Read the model definition and answer for the solid it produces. Units are mm, in the model's axes. Face numbers are marked on the shaded views. A direction names the side the tool comes from. Coordinates: 2 decimals unless noted, no trailing zeros. Loops run counter-clockwise (first coordinate to the right, second up) from the corner with the lowest first, then second, coordinate; pieces in that order, holes last.
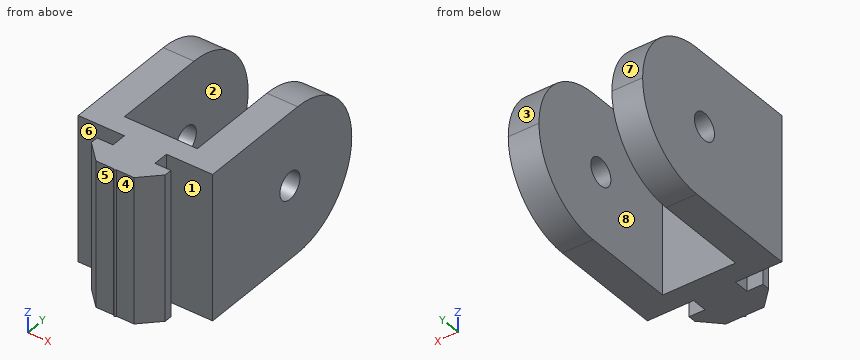
from build123d import *

# Parameters (mm, degrees)
SKETCH1_W           = 150
SKETCH1_H           = 70
BOSS_EXTRUDE1_DEPTH = 10
SKETCH2_W           = 18
SKETCH2_H           = 70
BOSS_EXTRUDE2_DEPTH = 80
FILLET1_R           = 35
SKETCH3_R           = 6.5
CUT_EXTRUDE1_DEPTH  = 164.102034121
RIB1_REACH          = 134.904
SKETCH5_WALL_W      = 321.142477346
SKETCH5_WALL_H      = 40
SKETCH7_W           = 43.830511012
SKETCH7_H           = 10.028409091
CUT_EXTRUDE2_DEPTH  = 80
SCALE1_SCALE        = 0.31
BOSS_EXTRUDE4_DEPTH = 21.7
CUT_EXTRUDE5_REACH  = 46.882
SKETCH11_W          = 1.005
SKETCH11_H          = 10.85
SKETCH11_H_2        = 13.95


with BuildPart() as part:
    # Sketch1 → Boss-Extrude1 (new body)
    with BuildSketch(Plane(origin=(0, 0, 0), x_dir=(1, 0, 0), z_dir=(0, 1, 0))):
        with Locations((14.225473782, -5.028409091)):
            Rectangle(SKETCH1_W, SKETCH1_H)
    extrude(amount=BOSS_EXTRUDE1_DEPTH)

    # Sketch2 → Boss-Extrude2 (add)
    with BuildSketch(Plane(origin=(0, 10, 0), x_dir=(1, 0, 0), z_dir=(0, 1, 0))):
        with Locations((-31.774526218, -5.028409091)):
            Rectangle(SKETCH2_W, SKETCH2_H)
        with Locations((21.225473782, -5.028409091)):
            Rectangle(SKETCH2_W, SKETCH2_H)
    extrude(amount=BOSS_EXTRUDE2_DEPTH)

    # Fillet1
    fillet1_edges = [part.edges().sort_by_distance(p)[0] for p in [
        (21.225473782, 90, 40.028409091),
        (21.225473782, 90, -29.971590909),
        (-31.774526218, 90, -29.971590909),
        (-31.774526218, 90, 40.028409091),
    ]]
    fillet(fillet1_edges, radius=FILLET1_R - 0.0001)  # a hair under: the kernel refuses the full size

    # Sketch3 → Cut-Extrude1 (cut, through all)
    with BuildSketch(Plane.ZY.offset(40.774526218)):
        with Locations((5.212032143, 50)):
            Circle(SKETCH3_R)
    extrude(amount=-CUT_EXTRUDE1_DEPTH, mode=Mode.SUBTRACT)

    # Sketch5 wall → Rib1 (add, up to next)
    with BuildSketch(Plane(origin=(52.140729288, 25.194278726, 0), x_dir=(0.821802771323, -0.569772064116, 0), z_dir=(0.569772064116, 0.821802771323, 0)), mode=Mode.PRIVATE) as rib1_sk1:
        Rectangle(SKETCH5_WALL_W, SKETCH5_WALL_H)
    rib1_tool1 = extrude(rib1_sk1.sketch, amount=-RIB1_REACH, mode=Mode.PRIVATE) - part.part
    add(rib1_tool1.solids().sort_by_distance((52.140729288, 25.194278726, 0))[0])

    # Sketch7 → Cut-Extrude2 (cut)
    with BuildSketch(Plane(origin=(0, 10, 0), x_dir=(1, 0, 0), z_dir=(0, 1, 0))):
        with Locations((52.140729288, 14.985795454)):
            Rectangle(SKETCH7_W, SKETCH7_H)
    extrude(amount=CUT_EXTRUDE2_DEPTH, mode=Mode.SUBTRACT)


with BuildPart() as part_1:
    # Scale1: scaled about (0, 0, 0)
    add(part.part.scale(SCALE1_SCALE))

    # Sketch10 → Boss-Extrude4 (add)
    with BuildSketch(Plane(origin=(0, 0, -9.291193182), x_dir=(-1, 0, 0), z_dir=(0, 0, -1))):
        Polygon((4.760103128, -1.455), (4.760103128, 0), (-1.489896872, 0), (-1.489896872, -1.455), (-1.489896872, -1.8), (-1.489896872, -2.3), (-3.864896872, -2.3), (-3.864896872, -3.439339828), (-1.204236701, -6.1), (1.425103128, -6.1), (1.635103128, -6.31), (1.845103128, -6.1), (4.474442956, -6.1), (7.135103128, -3.439339828), (7.135103128, -2.3), (4.760103128, -2.3), (4.760103128, -1.8), align=None)
    extrude(amount=-BOSS_EXTRUDE4_DEPTH)

    # Sketch11 → Cut-Extrude5 (cut, up to next)
    with BuildSketch(Plane(origin=(0, 0, -9.291193182), x_dir=(-1, 0, 0), z_dir=(0, 0, -1)), mode=Mode.PRIVATE) as cut_extrude5_sk1:
        Polygon((-9.369896872, 3.1), (-8.364896872, 3.1), (-8.364896872, 17.05), (-9.369896872, 17.05), (-9.369896872, 12.52045281), align=None)
    cut_extrude5_tool1 = extrude(cut_extrude5_sk1.sketch, amount=-CUT_EXTRUDE5_REACH, mode=Mode.PRIVATE) & part_1.part
    # Sketch11 → Cut-Extrude5 (cut, up to next)
    with BuildSketch(Plane(origin=(0, 0, -9.291193182), x_dir=(-1, 0, 0), z_dir=(0, 0, -1)), mode=Mode.PRIVATE) as cut_extrude5_sk2:
        with Locations((-8.867396872, 22.475)):
            Rectangle(SKETCH11_W, SKETCH11_H)
    cut_extrude5_tool2 = extrude(cut_extrude5_sk2.sketch, amount=-CUT_EXTRUDE5_REACH, mode=Mode.PRIVATE) & part_1.part
    # Sketch11 → Cut-Extrude5 (cut, up to next)
    with BuildSketch(Plane(origin=(0, 0, -9.291193182), x_dir=(-1, 0, 0), z_dir=(0, 0, -1)), mode=Mode.PRIVATE) as cut_extrude5_sk3:
        Polygon((-22.957355286, 3.1), (-9.369896872, 3.1), (-9.369896872, 12.52045281), align=None)
    cut_extrude5_tool3 = extrude(cut_extrude5_sk3.sketch, amount=-CUT_EXTRUDE5_REACH, mode=Mode.PRIVATE) & part_1.part
    # Sketch11 → Cut-Extrude5 (cut, up to next)
    with BuildSketch(Plane(origin=(0, 0, -9.291193182), x_dir=(-1, 0, 0), z_dir=(0, 0, -1)), mode=Mode.PRIVATE) as cut_extrude5_sk4:
        Polygon((-8.364896872, 0), (-8.364896872, 3.1), (-9.369896872, 3.1), (-22.957355286, 3.1), (-27.659896872, 3.1), (-27.659896872, 0), align=None)
    cut_extrude5_tool4 = extrude(cut_extrude5_sk4.sketch, amount=-CUT_EXTRUDE5_REACH, mode=Mode.PRIVATE) & part_1.part
    # Sketch11 → Cut-Extrude5 (cut, up to next)
    with BuildSketch(Plane(origin=(0, 0, -9.291193182), x_dir=(-1, 0, 0), z_dir=(0, 0, -1)), mode=Mode.PRIVATE) as cut_extrude5_sk5:
        with Locations((12.137603128, 10.075)):
            Rectangle(SKETCH11_W, SKETCH11_H_2)
    cut_extrude5_tool5 = extrude(cut_extrude5_sk5.sketch, amount=-CUT_EXTRUDE5_REACH, mode=Mode.PRIVATE) & part_1.part
    # Sketch11 → Cut-Extrude5 (cut, up to next)
    with BuildSketch(Plane(origin=(0, 0, -9.291193182), x_dir=(-1, 0, 0), z_dir=(0, 0, -1)), mode=Mode.PRIVATE) as cut_extrude5_sk6:
        with Locations((12.137603128, 22.475)):
            Rectangle(SKETCH11_W, SKETCH11_H)
    cut_extrude5_tool6 = extrude(cut_extrude5_sk6.sketch, amount=-CUT_EXTRUDE5_REACH, mode=Mode.PRIVATE) & part_1.part
    # Sketch11 → Cut-Extrude5 (cut, up to next)
    with BuildSketch(Plane(origin=(0, 0, -9.291193182), x_dir=(-1, 0, 0), z_dir=(0, 0, -1)), mode=Mode.PRIVATE) as cut_extrude5_sk7:
        Polygon((12.640103128, 3.1), (11.635103128, 3.1), (11.635103128, 0), (18.840103128, 0), (18.840103128, 3.1), align=None)
    cut_extrude5_tool7 = extrude(cut_extrude5_sk7.sketch, amount=-CUT_EXTRUDE5_REACH, mode=Mode.PRIVATE) & part_1.part
    add(cut_extrude5_tool1.solids().sort_by_distance((8.867397, 10.075, -9.291193))[0], mode=Mode.SUBTRACT)
    add(cut_extrude5_tool2.solids().sort_by_distance((8.867397, 22.475, -9.291193))[0], mode=Mode.SUBTRACT)
    add(cut_extrude5_tool3.solids().sort_by_distance((13.89905, 6.240151, -9.291193))[0], mode=Mode.SUBTRACT)
    add(cut_extrude5_tool4.solids().sort_by_distance((18.012397, 1.55, -9.291193))[0], mode=Mode.SUBTRACT)
    add(cut_extrude5_tool5.solids().sort_by_distance((-12.137603, 10.075, -9.291193))[0], mode=Mode.SUBTRACT)
    add(cut_extrude5_tool6.solids().sort_by_distance((-12.137603, 22.475, -9.291193))[0], mode=Mode.SUBTRACT)
    add(cut_extrude5_tool7.solids().sort_by_distance((-15.237603, 1.55, -9.291193))[0], mode=Mode.SUBTRACT)


solid = part_1.part
Q1. A cutting plane is placed at D-D (z = 7.75). Give the vertices of the cut face in (x, y).
Findings below:
outline: (-11.64, 0) - (-4.76, 0) - (-4.76, -2.3) - (-7.14, -2.3) - (-7.14, -3.44) - (-4.47, -6.1) - (-1.85, -6.1) - (-1.64, -6.31) - (-1.43, -6.1) - (1.2, -6.1) - (3.86, -3.44) - (3.86, -2.3) - (1.49, -2.3) - (1.49, 0) - (8.36, 0) - (8.36, 25.96) - (3.79, 25.96) - (3.79, 3.1) - (-7.06, 3.1) - (-7.06, 25.96) - (-11.64, 25.96) - close
Q2. A cutting plane is placed at B-B (y = 6). Give the vertices of the cut face in (x, z), then the cut area to 3 significant figures.
Findings below:
outline: (-11.64, -9.29) - (-7.06, -9.29) - (-7.06, 12.41) - (-11.64, 12.41) - close; (3.79, -9.29) - (8.36, -9.29) - (8.36, 12.41) - (3.79, 12.41) - close
area: 199 mm2
Q3. Which of the six approach directions +Z, -Z, +X, -X, +Y, -Y give full straight-line access (tool end or side, diameter ignored) to the marked faces 1, 2, 3, 4 and 5?
Findings below:
face 1: +Z, -Z, +X
face 2: +Z, -Z, +Y
face 3: +Z, +X, -X, +Y
face 4: +Z, -Z, +X, -Y
face 5: +Z, -Z, -X, -Y
Q4. Straight lines are drawn through the part: probe 1 along X at (y, z) = (8, 9.75); probe 2 along X at (y, z) = (-2, 2); probe 3 along Y at (x, z) = (-5, -3.75). For each, find the intervals that lie inside material, in ascending order.
Findings below:
probe 1: x = -11.64 to -7.06, 3.79 to 8.36
probe 2: x = -4.76 to 1.49
probe 3: y = -5.57 to -2.3, 0 to 3.1
Q5. A cutting plane is placed at A-A (y = 15.5). Give the vertices of the cut face in (x, z).
Findings below:
outline: (-11.64, -9.29) - (-7.06, -9.29) - (-7.06, -0.4) - (-11.64, -0.4) - close; (-11.64, 3.63) - (-7.06, 3.63) - (-7.06, 12.41) - (-11.64, 12.41) - close; (3.79, -9.29) - (8.36, -9.29) - (8.36, -0.4) - (3.79, -0.4) - close; (3.79, 3.63) - (8.36, 3.63) - (8.36, 12.41) - (3.79, 12.41) - close
Q6. Flat-ended cylindrical pins translate along their axes: pin 1 Ø1.2 at (x, z) = (-5.5, 1.5) entering from +Y; pin 2 Ø6 at (y, z) = (-2, 5.5) entering from -X; pin 3 Ø0.8 at (x, z) = (0.5, -1) entering from -Y; pin 4 Ø1.2 at (y, z) = (-1, -3.5) entering from -X. Find the tip coordinate at first contact, or state that the pin passes through.
Findings below:
pin 1: stops at y = 3.1
pin 2: stops at x = -11.64
pin 3: stops at y = -6.1
pin 4: stops at x = -4.76
Q7. Determine the mould class of the marked faces 6, 7 and 8 for opening direction Y: +Y half, -Y half, draft (parallel to the pull), parting line (faces both ways), or undercut.
Findings below:
face 6: undercut
face 7: +Y half
face 8: draft
